Check sheet for the modelled part. Datum: model origin and axes. Units: mm. A direction names the side the tool comes from. Round coordinates to 2 decimals unless told otherwise and drop trailing zeros. Order: outer loops, then holes, each group sorted by start corner. A loop starts at its lowest first (then second) coordinate and runs counter-clockwise, first axis right, second up.
(1) Thickness scan on probe 1 along X at (y, z) = (1.6, 15); probe 2 along X at (y, z) = (2.55, -13); probe 3 along X at (y, z) = (1.1, 10). Record the ranges inside material, lowest first.
(2) Sectioned sample at C-C, the plane z = 9.5. Enter the section's corners in (x, y) (3 decimals), and give its area (3 significant figures).
(3) Tool access check on faces 4 (the cylindrical face through (-45.77, 1.61, -13.87)), 5 (the flat face through (46, 2, 7.747)), 6 (the flat face through (-41.148, 2, 13)). Record the directions out of +Z, -Z, +X, -X, +Y, -Y that give a thin tool (end or side, any length) a straight path to the whole face; none if there is none.
(4) Sectioned sample at B-B, the plane y = 2.6. Count the separate pieces of the cut face and the enclosed holes in it, and give its area (3 significant figures).
(5) Mould release check, pull along X, two halves, no side actions. Record for faces 1 (the cylindrical face through (36.522, 1.61, -11.105)), 2 (the flat face through (-1, 2, 17.907)), 3 (the flat face through (41.148, 2, 13)): released by +X, released by -X, zero draft, split by the parting line, or undercut.
(6) Depth check by flat-ended pin: pin 1 (6 mm diameter, centred on x = -37.973, z = 14.732, fed in from -Y); pin 2 (3 mm diameter, centred on x = 47.625, z = -14.986, fed in from +Y); pin 3 (1.6 mm diameter, centred on x = -47.5, y = 1.5, fed in from +Z). Enter the tip coordinate at first touch or a pass-through.
(7) Sectioned sample at A-A, the plane x = -37.5. Enter the section's corners in (y, z) (3 decimals), and give its area (3 significant figures).
```python
from build123d import *

# Parameters (mm, degrees)
SKETCH2_W           = 101.6
SKETCH2_H           = 35.814
BOSS_EXTRUDE1_DEPTH = 3.175
SKETCH3_R           = 1.8288
CUT_EXTRUDE1_DEPTH  = 4.175
SKETCH4_R           = 1.8288
CUT_EXTRUDE2_DEPTH  = 4.175
SKETCH5_W           = 9.651618186
SKETCH5_H           = 10.16
CUT_EXTRUDE3_DEPTH  = 4.175


with BuildPart() as part:
    # Sketch2 → Boss-Extrude1 (new body)
    with BuildSketch(Plane(origin=(0, 0, 0), x_dir=(1, 0, 0), z_dir=(0, 1, 0))):
        Rectangle(SKETCH2_W, SKETCH2_H)
    extrude(amount=BOSS_EXTRUDE1_DEPTH)

    # Sketch3 → Cut-Extrude1 (cut, through all)
    with BuildSketch(Plane(origin=(0, 3.175, 0), x_dir=(1, 0, 0), z_dir=(0, 1, 0))):
        with Locations((47.625, 14.986)):
            Circle(SKETCH3_R)
        with Locations((47.625, -4.572)):
            Circle(SKETCH3_R)
        with Locations((-44.323, 14.986)):
            Circle(SKETCH3_R)
        with Locations((-44.323, -4.572)):
            Circle(SKETCH3_R)
    extrude(amount=-CUT_EXTRUDE1_DEPTH, mode=Mode.SUBTRACT)

    # Sketch4 → Cut-Extrude2 (cut, through all)
    with BuildSketch(Plane(origin=(0, 3.175, 0), x_dir=(1, 0, 0), z_dir=(0, 1, 0))):
        with Locations((-37.973, -14.732)):
            Circle(SKETCH4_R)
        with Locations((-37.973, 12.2174)):
            Circle(SKETCH4_R)
        with Locations((37.973, -14.732)):
            Circle(SKETCH4_R)
        with Locations((37.973, 12.2174)):
            Circle(SKETCH4_R)
    extrude(amount=-CUT_EXTRUDE2_DEPTH, mode=Mode.SUBTRACT)

    # Sketch5 → Cut-Extrude3 (cut, through all)
    with BuildSketch(Plane(origin=(0, 3.175, 0), x_dir=(1, 0, 0), z_dir=(0, 1, 0))):
        with Locations((45.974190907, -12.827)):
            Rectangle(SKETCH5_W, SKETCH5_H)
        with Locations((-45.974190907, -12.827)):
            Rectangle(SKETCH5_W, SKETCH5_H)
    extrude(amount=-CUT_EXTRUDE3_DEPTH, mode=Mode.SUBTRACT)


solid = part.part
```
Derived:
1. probe 1: x = -41.15 to -39.78, -36.16 to 36.16, 39.78 to 41.15
1. probe 2: x = -50.8 to -39.63, -36.32 to 36.32, 39.63 to 50.8
1. probe 3: x = -41.15 to 41.15
2. outline: (-41.148, 0) - (41.148, 0) - (41.148, 3.175) - (-41.148, 3.175) - close
2. area: 261 mm2
3. face 4: +Y, -Y
3. face 5: +Z, +X, +Y, -Y
3. face 6: +Z, -X, +Y, -Y
4. separate pieces: 1
4. enclosed holes: 8
4. area: 3,360 mm2
5. face 1: undercut
5. face 2: zero draft
5. face 3: released by +X
6. pin 1: stops at y = 0
6. pin 2: passes through
6. pin 3: stops at z = 7.75
7. outline: (0, -17.907) - (3.175, -17.907) - (3.175, -13.984) - (0, -13.984) - close; (0, -10.451) - (3.175, -10.451) - (3.175, 12.965) - (0, 12.965) - close; (0, 16.499) - (3.175, 16.499) - (3.175, 17.907) - (0, 17.907) - close
7. area: 91.3 mm2
